Input: part model. Units: mm. Frame: model coordinates. A direction names the side the tool comes from. Coordinates: 2 decimals unless noted, no trailing zeros. Loops run counter-clockwise (first coordinate to the right, second up) from the corner with the lowest first, then second, coordinate; pieces in that order, holes last. Notation, with made-up numbers: (28, 14) - (35, 14) arc R17 cw to (35, 42) - close; hole circle Ø11 at (37.25, 0.25). An arc over 180 degrees is marked (long way). Use one line per item in the form item = value.
from build123d import *

# Parameters (mm, degrees)
F0_R            = 45
F1_DEPTH        = 6
F2_R            = 3.25
F3_DEPTH        = 12.5
F3_COPIES_COUNT = 6


# Not quite as in the source:
# - a pattern or mirror of a feature is missing from the dataset's text; its kind, count and spacing are read off the source's solid


with BuildPart() as f1:
    # F0 (on Front) → F1 (new body)
    with BuildSketch(Plane.XZ):
        Circle(F0_R)
        Polygon((-21.0098581772, 21.0098581772), (-7.6901418228, 28.7), (7.6901418228, 28.7), (21.0098581772, 21.0098581772), (28.7, 7.6901418228), (28.7, -7.6901418228), (21.0098581772, -21.0098581772), (7.6901418228, -28.7), (-7.6901418228, -28.7), (-21.0098581772, -21.0098581772), (-28.7, -7.6901418228), (-28.7, 7.6901418228), align=None, mode=Mode.SUBTRACT)
    extrude(amount=F1_DEPTH)

    # F2 (on face) → F3 (cut, symmetric)
    with BuildSketch(Plane.XZ.offset(6)):
        with Locations((0, 37)):
            Circle(F2_R)
    f3 = extrude(amount=F3_DEPTH, both=True, mode=Mode.SUBTRACT)

    # F3_copies: F3 ×6 about axis
    f3_copies_axis = Axis((0, 0, 0), (0, 1, 0))
    for i in range(1, F3_COPIES_COUNT):
        add(f3.rotate(f3_copies_axis, i * 360 / F3_COPIES_COUNT), mode=Mode.SUBTRACT)


solid = f1.part
Q1. Cut plane C-C, the plane z = -18.5. Return loops of the section in (x, y).
Check values:
outline = (-41.02, -6) - (-35.29, -6) - (-35.29, 0) - (-41.02, 0) - close; (-28.79, -6) - (-22.46, -6) - (-22.46, 0) - (-28.79, 0) - close; (22.46, -6) - (28.79, -6) - (28.79, 0) - (22.46, 0) - close; (35.29, -6) - (41.02, -6) - (41.02, 0) - (35.29, 0) - close
Q2. Ray query, line 1 along Z through (x, y) = (0, -3.2); line 2 along X through (y, z) = (-1.05, 21); line 3 along Z through (x, y) = (29.5, -4). Return the intervals inside material, ascending. Write a range as [from, to].
Check values:
line_1 = [-45, -40.25], [-33.75, -28.7], [28.7, 33.75], [40.25, 45]
line_2 = [-39.8, -34.12], [-29.97, -21.02], [21.02, 29.97], [34.12, 39.8]
line_3 = [-33.98, -20.52], [-16.48, 16.48], [20.52, 33.98]
Q3. First-contact query: P1, Ø1, axis at y = -2.5, z = -25.5, coming from the +X side; P2, Ø6, axis at x = 7.5, z = 24, coming from the -Y side; P3, Ø3, axis at x = -19.5, y = -5, coming from the +Z side. Flat tips, straight axial feed; report the tip coordinate or a pass-through.
Check values:
P1 = 37.42
P2 = through
P3 = 41.24
Q4. Cut plane D-D, the plane x = -16.5. Return loops of the section in (y, z).
Check values:
outline = (-6, -41.87) - (0, -41.87) - (0, -23.61) - (-6, -23.61) - close; (-6, 23.61) - (0, 23.61) - (0, 41.87) - (-6, 41.87) - close
Q5. Cut plane A-A, the plane x = 0. Return loops of the section in (y, z).
Check values:
outline = (-6, -45) - (0, -45) - (0, -40.25) - (-6, -40.25) - close; (-6, -33.75) - (0, -33.75) - (0, -28.7) - (-6, -28.7) - close; (-6, 28.7) - (0, 28.7) - (0, 33.75) - (-6, 33.75) - close; (-6, 40.25) - (0, 40.25) - (0, 45) - (-6, 45) - close
Q6. Cut plane B-B, the plane y = -4.5. Return loops of the section in (x, z), then the cut area to 3 significant figures.
Check values:
outline = circle Ø90 at (0, 0); hole circle Ø6.5 at (-32.04, -18.5); hole circle Ø6.5 at (-32.04, 18.5); hole (-28.7, -7.69) - (-21.01, -21.01) - (-7.69, -28.7) - (7.69, -28.7) - (21.01, -21.01) - (28.7, -7.69) - (28.7, 7.69) - (21.01, 21.01) - (7.69, 28.7) - (-7.69, 28.7) - (-21.01, 21.01) - (-28.7, 7.69) - close; hole circle Ø6.5 at (0, -37); hole circle Ø6.5 at (0, 37); hole circle Ø6.5 at (32.04, -18.5); hole circle Ø6.5 at (32.04, 18.5)
area = 3,510 mm²
Q7. Set-up query: faces 1 (the flat face through (29, -6, 1)), 2 (the flat face through (24.909, -2.958, -14.257)). Return all of +Z, -Z, +X, -X, +Y, -Y with unobstructed straight access to the full face (end or side cutting, diameter ignored); none if empty.
Check values:
face_1 = +Z, -Z, +X, -X, -Y
face_2 = +Y, -Y
Q8. Pull-direction query (X, two-part tool) for faces 3 (the cylindrical face through (29.464, -3.042, -20.478)), 4 (the flat face through (29, 0, 1)); classes: pulls with the +X half, pulls with the -X half, needs draft (parallel to the pull), parting line crosses it, or undercut.
Check values:
face_3 = undercut
face_4 = needs draft
